from build123d import *

# Parameters (mm, degrees)
SKETCH1_W           = 25.4
SKETCH1_H           = 25.4
SKETCH1_W_2         = 20.32
SKETCH1_H_2         = 20.32
EXTRUDE_THIN1_DEPTH = 189.58179
SKETCH2_R           = 2.4892
CUT_EXTRUDE1_DEPTH  = 26.4


with BuildPart() as part:
    # Sketch1 → Extrude-Thin1 (new body, symmetric)
    with BuildSketch(Plane.XY):
        with Locations((12.7, 12.7)):
            Rectangle(SKETCH1_W, SKETCH1_H)
        with Locations((12.7, 12.7)):
            Rectangle(SKETCH1_W_2, SKETCH1_H_2, mode=Mode.SUBTRACT)
    extrude(amount=EXTRUDE_THIN1_DEPTH, both=True)

    # Sketch2 → Cut-Extrude1 (cut, through all)
    with BuildSketch(Plane(origin=(0, 25.4, 0), x_dir=(1, 0, 0), z_dir=(0, 1, 0))):
        with Locations((12.7, -176.88179)):
            Circle(SKETCH2_R)
        with Locations((12.7, -151.48179)):
            Circle(SKETCH2_R)
        with Locations((12.7, 176.88179)):
            Circle(SKETCH2_R)
        with Locations((12.7, 151.48179)):
            Circle(SKETCH2_R)
    extrude(amount=-CUT_EXTRUDE1_DEPTH, mode=Mode.SUBTRACT)


solid = part.part
Work out the finished part from the listing and answer in its coordinate system (mm). A direction names the side the tool comes from. Round coordinates to 2 decimals unless told otherwise and drop trailing zeros. Loops run counter-clockwise (first coordinate to the right, second up) from the corner with the lowest first, then second, coordinate; pieces in that order, holes last. Notation, with made-up numbers: (20.25, 46.25) - (31.25, 46.25) arc R23 ccw to (31.25, 63.25) - close; hole circle Ø7 at (-22, 84.25). An arc over 180 degrees is marked (long way). Use one line per item in the form item = value. Start each with the question number.
(1) Consider line 1 (Z direction, x = 12.7, y = 1.65); line 2 (Y direction, x = 21.25, z = -30.5). Determine where each line is inside the solid, lowest interval first.
(2) A flat-ended cylindrical pin translates along its axis: P1, Ø4, axis at x = 12.7, z = 176.88, coming from the +Y side. Find the tip coordinate at first contact, or state that the pin passes through.
(3) Find section A-A on y = 5.75. Determine the outline of the cut face in (x, z).
(4) Determine the mould class of faces 1 (the face through (13, 22.86, 3)), 2 (the face through (13, 25.4, 3)), 3 (the face through (0, 13, 3)), 4 (the face through (25.4, 13, 3)) for opening direction X: +X half, -X half, draft (parallel to the pull), parting line (faces both ways), or undercut.
(5) Find section B-B on z = 75. Determine the outline of the cut face in (x, y).
(6) Which of the six approach directions +Z, -Z, +X, -X, +Y, -Y give full straight-line access (tool end or side, diameter ignored) to faces 5 (the face through (24, 13, -189.582)), 6 (the face through (2.54, 13, 3))?
Answer list:
q1.line_1 = -189.58 to -179.37, -174.39 to -153.97, -148.99 to 148.99, 153.97 to 174.39, 179.37 to 189.58
q1.line_2 = 0 to 2.54, 22.86 to 25.4
q2.P1 = through
q3.outline = (0, -189.58) - (2.54, -189.58) - (2.54, 189.58) - (0, 189.58) - close; (22.86, -189.58) - (25.4, -189.58) - (25.4, 189.58) - (22.86, 189.58) - close
q4.face_1 = undercut
q4.face_2 = draft
q4.face_3 = -X half
q4.face_4 = +X half
q5.outline = (0, 0) - (25.4, 0) - (25.4, 25.4) - (0, 25.4) - close; hole (2.54, 2.54) - (22.86, 2.54) - (22.86, 22.86) - (2.54, 22.86) - close
q6.face_5 = -Z, +X, -X, +Y, -Y
q6.face_6 = +Z, -Z
